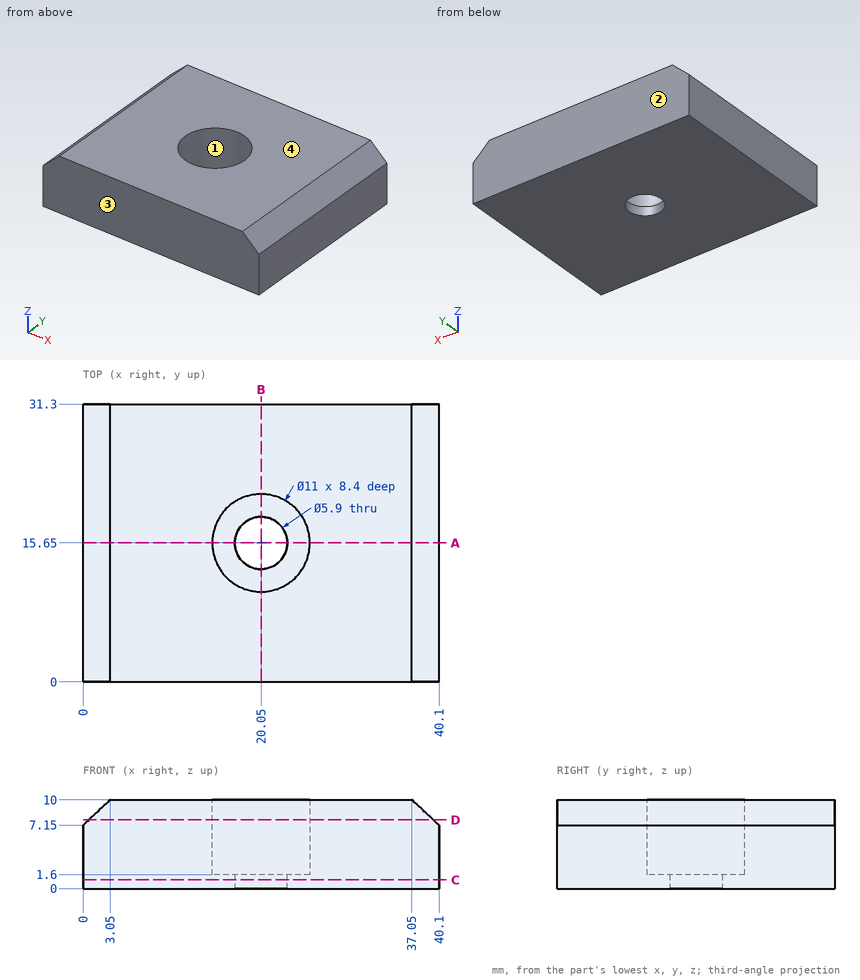
Can you work these out from the drawing? Everything is in mm from the part's minimum corner. Round coordinates to 2 decimals unless told otherwise and drop trailing zeros. Order: outer loops, then holes, each group sorted by start corner. A loop starts at its lowest first (then second) coordinate and runs counter-clockwise, first axis right, second up. Notation, with made-up numbers: M -25,-28.5 L -11,-28.5 A32 ccw -11,6.5 Z; hole C 27.25,38.5 d8. An arc over 180 degrees is marked long. Answer as CSV lines item,"result".
Item 1: Please list where these lines run through material, in increasing order: L1, parallel to Y at x = 20.05, z = 0.55; L2, parallel to X at y = 15.65, z = 0.5; L3, parallel to Y at x = 20.05, z = 7. Write a range as [from, to].
From the geometry:
L1,"[0, 12.7], [18.6, 31.3]"
L2,"[0, 17.1], [23, 40.1]"
L3,"[0, 10.15], [21.15, 31.3]"
Item 2: Imagine slicing it at D-D on z = 7.75. List the corners of the cut face in (x, y) for me, and give its area (3 significant figures).
From the geometry:
outline,"M 0.64,0 L 39.46,0 L 39.46,31.3 L 0.64,31.3 Z; hole C 20.05,15.65 d11"
area,"1,120 mm2"
Item 3: We'd pull the mould along Y, two halves only. Please class the marked faces 1, 2, 3 and 4: +Y half, -Y half, draft (parallel to the pull), parting line (faces both ways), or undercut.
From the geometry:
face 1,"undercut"
face 2,"+Y half"
face 3,"-Y half"
face 4,"draft"
Item 4: Imagine slicing it at C-C on z = 1. List the corners of the cut face in (x, y) for me, and give its area (3 significant figures).
From the geometry:
outline,"M 0,0 L 40.1,0 L 40.1,31.3 L 0,31.3 Z; hole C 20.05,15.65 d5.9"
area,"1,230 mm2"
Item 5: Imagine slicing it at A-A on y = 15.65. List the corners of the cut face in (x, z) for me.
From the geometry:
outline,"M 0,0 L 17.1,0 L 17.1,1.6 L 14.55,1.6 L 14.55,10 L 3.05,10 L 0,7.15 Z; M 23,0 L 40.1,0 L 40.1,7.15 L 37.05,10 L 25.55,10 L 25.55,1.6 L 23,1.6 Z"
Item 6: Imagine slicing it at B-B on x = 20.05. List the corners of the cut face in (y, z) for me.
From the geometry:
outline,"M 0,0 L 12.7,0 L 12.7,1.6 L 10.15,1.6 L 10.15,10 L 0,10 Z; M 18.6,0 L 31.3,0 L 31.3,10 L 21.15,10 L 21.15,1.6 L 18.6,1.6 Z"
Item 7: For pin 1 (7.5 mm diameter, centred on x = 20.05, y = 15.65, fed in from +Z), with a flat end and sliding along its axis, tell me the tip position at first contact or that it passes through.
From the geometry:
pin 1,"z = 1.6"
